```python
from build123d import *

# Parameters (mm, degrees)
F1_DEPTH = 10
F2_R     = 5
F3_R     = 1.5


with BuildPart() as f1:
    # F0 (on Top) → F1 (new body)
    with BuildSketch(Plane.XY):
        with BuildLine():
            Line((86.928109, 22.5), (-90, 22.5))
            ThreePointArc((-90, 22.5), (-112.5, 0), (-90, -22.5))
            Line((-90, -22.5), (86.879614, -22.5))
            ThreePointArc((86.879614, -22.5), (116.008795, -39.840686), (147.998941, -28.622881))
            Line((147.998941, -28.622881), (129.205089, -21.782478))
            Line((129.205089, -21.782478), (125.732125, -2.086323))
            Line((125.732125, -2.086323), (141.053014, 10.769429))
            Line((141.053014, 10.769429), (159.805062, 3.944242))
            ThreePointArc((159.805062, 3.944242), (129.869799, 38.763218), (86.928109, 22.5))
        make_face()
    extrude(amount=F1_DEPTH)

    # F2
    f2_edges = [f1.edges().sort_by_distance(p)[0] for p in [
        (86.928109, 22.5, 5),
        (86.879614, -22.5, 5),
    ]]
    fillet(f2_edges, radius=F2_R)

    # F3
    f3_edges = [f1.edges().sort_by_distance(p)[0] for p in [
        (-2.809759, 22.5, 10),
        (-2.835085, -22.5, 0),
    ]]
    fillet(f3_edges, radius=F3_R)


solid = f1.part
```
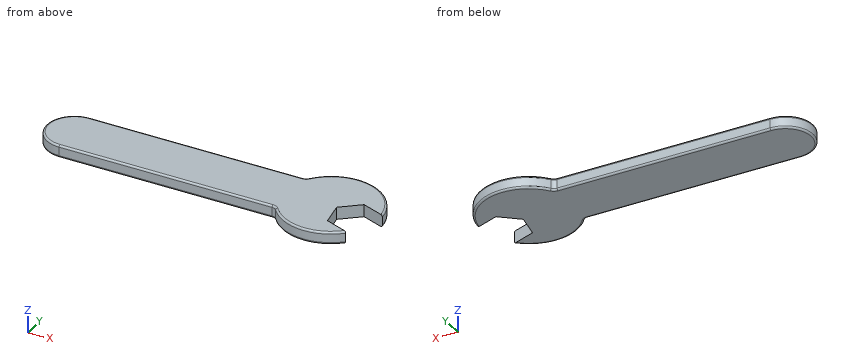
Design review of the part built by this model. Coordinates are the model's own, in mm. Give positions to 0.01 mm unless a question says otherwise; leave off trailing zeros. Loops run counter-clockwise (first coordinate to the right, second up) from the corner with the lowest first, then second, coordinate; pieces in that order, holes last. Notation, with made-up numbers: (61.25, 33) -> (66.25, 33) arc R16 cw to (66.25, 45) -> close; hole circle Ø8 at (-20, 33.5). An arc over 180 degrees is marked (long way). Write each question's results on one line, items separated by ' | '.
Q1. Take a section at B-B, the plane x = 3. Write out the cut boundary in (y, z), plus the area to 3 significant figures.
Reply:
outline: (-22.5, 1.5) arc R1.5 ccw to (-21, 0) -> (21, 0) arc R1.5 ccw to (22.5, 1.5) -> (22.5, 8.5) arc R1.5 ccw to (21, 10) -> (-21, 10) arc R1.5 ccw to (-22.5, 8.5) -> close | area: 448 mm²
Q2. Wall thickness on L1, parallel to Y at x = -82, z = 1.5; L2, parallel to X at y = 17.5, z = 8; L3, parallel to X at y = 12, z = 8: over which ranges is each line inside the solid? List them lowest first.
Reply:
L1: y = -22.5 to 22.5 | L2: x = -104.14 to 155.97 | L3: x = -109.03 to 158.16
Q3. For pin 1 Ø4 at (x, z) = (125, 9) entering from -Y; pin 2 Ø1 at (x, z) = (76, 3.5) entering from -Y; pin 3 Ø5.5 at (x, z) = (26.5, 4) entering from +Y, all flat-tipped, find the tip position at first contact; note any pin that passes through.
Reply:
pin 1: stops at y = -39.92 | pin 2: stops at y = -22.5 | pin 3: stops at y = 22.5
Q4. Take a section at A-A, the plane z = 3.5. Write out the cut boundary in (x, y), plus the area to 3 significant figures.
Reply:
outline: (-90, -22.5) -> (84.33, -22.5) arc R5 cw to (88.29, -24.45) arc R40.04 ccw to (148, -28.62) -> (129.21, -21.78) -> (125.73, -2.09) -> (141.05, 10.77) -> (159.81, 3.94) arc R40 ccw to (88.34, 24.44) arc R5 cw to (84.38, 22.5) -> (-90, 22.5) arc R22.5 ccw to start | area: 12,600 mm²
